The model under review builds one solid part; all positions refer to its coordinate system, in mm. Round coordinates to 2 decimals unless told otherwise and drop trailing zeros. Loops run counter-clockwise (first coordinate to the right, second up) from the corner with the lowest first, then second, coordinate; pieces in that order, holes last. Notation, with made-up numbers: (80.25, 6.5) -> (101.25, 6.5) arc R17 ccw to (101.25, 19.5) -> close; hole circle Ø9 at (-39.75, 27). An arc over 180 degrees is marked (long way). Write each question's results on one line, items separated by ' | '. Start each with the question number.
Item 1: For L1, parallel to Z at x = -3.25, y = 0; L2, parallel to Z at x = 0, y = 3.5; L3, parallel to Y at x = 0, z = 5.5 (3 decimals), list the stretches that pass through material, from the lowest coordinate up. Write a range as from..to.
Item 2: Clearance check with flat-ended pins moving along their axes: pin 1 Ø1 at (x, z) = (-1.5, -32.5) entering from -Y; pin 2 Ø3 at (x, z) = (-0.5, -41) entering from -Y (3 decimals); pin 3 Ø0.8 at (y, z) = (0.5, 22.5) entering from +X. State where each tip first meets the part, or that it passes through.
Item 3: We need section B-B (y = 0). Give the boundary of the cut face in (x, z) (1 decimal).
Item 4: We need section A-A (x = 0). Give the boundary of the cut face in (y, z) (1 decimal).
Item 5: We need section C-C (z = -14). Give the boundary of the cut face in (x, y) (3 decimals).
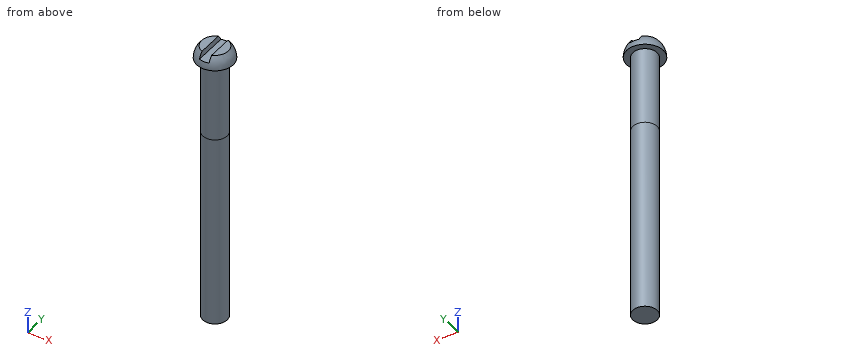
from build123d import *

# Parameters (mm, degrees)
SKETCH1_R               = 3.175
BOSS_EXTRUDE1_DEPTH     = 20.32
REVOLVE1_ANGLE          = 180
CUT_EXTRUDE1_DEPTH      = 8.382
CUT_EXTRUDE1_DEPTH_BACK = 9.398
SKETCH3_W               = 1.756055425
SKETCH3_H               = 11.721669961
SKETCH4_W               = 2.54
SKETCH4_H               = 12.81199514
CUT_EXTRUDE2_DEPTH      = 1.524
BOSS_EXTRUDE2_START     = 50.8
SKETCH5_R               = 3.175
BOSS_EXTRUDE2_DEPTH     = 50.8


with BuildPart() as part:
    # Sketch1 → Boss-Extrude1 (new body)
    with BuildSketch(Plane.XY):
        Circle(SKETCH1_R)
    extrude(amount=BOSS_EXTRUDE1_DEPTH)

    # Sketch2 → Revolve1 (revolve)
    with BuildSketch(Plane.XY.offset(20.32)):
        with BuildLine():
            Line((0, -4.7625), (0, 4.7625))
            ThreePointArc((0, 4.7625), (4.7625, 0), (0, -4.7625))
        make_face()
    revolve(axis=Axis((0, -4.7625, 20.32), (0, -1, 0)), revolution_arc=REVOLVE1_ANGLE)

    # Sketch3 → Cut-Extrude1 (cut, two sides: drawn at the far end of the back side and taken through both)
    with BuildSketch(Plane(origin=(2.54, 0, 0), x_dir=(0, 0, -1), z_dir=(1, 0, 0)).offset(-CUT_EXTRUDE1_DEPTH_BACK)):
        with Locations((-24.463510257, -1.014387128)):
            Rectangle(SKETCH3_W, SKETCH3_H)
    extrude(amount=CUT_EXTRUDE1_DEPTH + CUT_EXTRUDE1_DEPTH_BACK, mode=Mode.SUBTRACT)

    # Sketch4 → Cut-Extrude2 (cut)
    with BuildSketch(Plane.XY.offset(23.585482544)):
        with Locations((0, -0.792879604)):
            Rectangle(SKETCH4_W, SKETCH4_H)
    extrude(amount=-CUT_EXTRUDE2_DEPTH, mode=Mode.SUBTRACT)

    # Sketch5 → Boss-Extrude2 (add)
    with BuildSketch(Plane(origin=(0, 0, 0), x_dir=(-1, 0, 0), z_dir=(0, 0, -1)).offset(BOSS_EXTRUDE2_START)):
        Circle(SKETCH5_R)
    extrude(amount=-BOSS_EXTRUDE2_DEPTH)


solid = part.part
Here are the results:
1) L1: z = 20.32..23.59 | L2: z = 20.32..22.06 | L3: y = -3.175..3.175
2) pin 1: stops at y = -3.01 | pin 2: stops at y = -3.175 | pin 3: stops at x = 4.39
3) outline: (-4.8, 20.3) -> (-3.2, 20.3) -> (-3.2, -50.8) -> (3.2, -50.8) -> (3.2, 20.3) -> (4.8, 20.3) arc R4.8 ccw to (3.5, 23.6) -> (1.3, 23.6) -> (1.3, 22.1) -> (-1.3, 22.1) -> (-1.3, 23.6) -> (-3.5, 23.6) arc R4.8 ccw to start
4) outline: (-4.8, 20.3) -> (-3.2, 20.3) -> (-3.2, -50.8) -> (3.2, -50.8) -> (3.2, 20.3) -> (4.8, 20.3) arc R4.8 ccw to (4.4, 22.1) -> (-4.4, 22.1) arc R4.8 ccw to start
5) outline: circle Ø6.35 at (0, 0)
